from build123d import *

# Parameters (mm, degrees)
SKETCH1_W           = 60
SKETCH1_H           = 160
SKETCH1_R           = 10
SKETCH1_R_2         = 10.5
BOSS_EXTRUDE1_DEPTH = 12
CUT_EXTRUDE1_REACH  = 88.279
SKETCH2_R           = 4
CUT_EXTRUDE2_REACH  = 102.717
SKETCH3_R           = 3


with BuildPart() as part:
    # Sketch1 → Boss-Extrude1 (new body)
    with BuildSketch(Plane(origin=(0, 0, 0), x_dir=(1, 0, 0), z_dir=(0, 1, 0))):
        Rectangle(SKETCH1_W, SKETCH1_H)
        with Locations(Location((0, 0, 0), (0, 0, 270))):
            Circle(SKETCH1_R, mode=Mode.SUBTRACT)
        with Locations(Location((0, 40, 0), (0, 0, 270))):
            Circle(SKETCH1_R_2, mode=Mode.SUBTRACT)
        with Locations(Location((0, -40, 0), (0, 0, 270))):
            Circle(SKETCH1_R_2, mode=Mode.SUBTRACT)
    extrude(amount=BOSS_EXTRUDE1_DEPTH)

    # Sketch2 → Cut-Extrude1 (cut, up to next)
    with BuildSketch(Plane(origin=(0, 12, 0), x_dir=(1, 0, 0), z_dir=(0, 1, 0)), mode=Mode.PRIVATE) as cut_extrude1_sk1:
        with Locations(Location((18, 50, 0), (0, 0, 270))):
            Circle(SKETCH2_R)
    cut_extrude1_tool1 = extrude(cut_extrude1_sk1.sketch, amount=-CUT_EXTRUDE1_REACH, mode=Mode.PRIVATE) & part.part
    # Sketch2 → Cut-Extrude1 (cut, up to next)
    with BuildSketch(Plane(origin=(0, 12, 0), x_dir=(1, 0, 0), z_dir=(0, 1, 0)), mode=Mode.PRIVATE) as cut_extrude1_sk2:
        with Locations(Location((18, -50, 0), (0, 0, 270))):
            Circle(SKETCH2_R)
    cut_extrude1_tool2 = extrude(cut_extrude1_sk2.sketch, amount=-CUT_EXTRUDE1_REACH, mode=Mode.PRIVATE) & part.part
    # Sketch2 → Cut-Extrude1 (cut, up to next)
    with BuildSketch(Plane(origin=(0, 12, 0), x_dir=(1, 0, 0), z_dir=(0, 1, 0)), mode=Mode.PRIVATE) as cut_extrude1_sk3:
        with Locations(Location((18, -20, 0), (0, 0, 270))):
            Circle(SKETCH2_R)
    cut_extrude1_tool3 = extrude(cut_extrude1_sk3.sketch, amount=-CUT_EXTRUDE1_REACH, mode=Mode.PRIVATE) & part.part
    # Sketch2 → Cut-Extrude1 (cut, up to next)
    with BuildSketch(Plane(origin=(0, 12, 0), x_dir=(1, 0, 0), z_dir=(0, 1, 0)), mode=Mode.PRIVATE) as cut_extrude1_sk4:
        with Locations(Location((18, 20, 0), (0, 0, 270))):
            Circle(SKETCH2_R)
    cut_extrude1_tool4 = extrude(cut_extrude1_sk4.sketch, amount=-CUT_EXTRUDE1_REACH, mode=Mode.PRIVATE) & part.part
    add(cut_extrude1_tool1.solids().sort_by_distance((18, 12, -50))[0], mode=Mode.SUBTRACT)
    add(cut_extrude1_tool2.solids().sort_by_distance((18, 12, 50))[0], mode=Mode.SUBTRACT)
    add(cut_extrude1_tool3.solids().sort_by_distance((18, 12, 20))[0], mode=Mode.SUBTRACT)
    add(cut_extrude1_tool4.solids().sort_by_distance((18, 12, -20))[0], mode=Mode.SUBTRACT)

    # Sketch3 → Cut-Extrude2 (cut, up to next)
    with BuildSketch(Plane(origin=(30, 0, 0), x_dir=(0, 0, -1), z_dir=(1, 0, 0)), mode=Mode.PRIVATE) as cut_extrude2_sk1:
        with Locations((50, 6)):
            Circle(SKETCH3_R)
    cut_extrude2_tool1 = extrude(cut_extrude2_sk1.sketch, amount=-CUT_EXTRUDE2_REACH, mode=Mode.PRIVATE) & part.part
    # Sketch3 → Cut-Extrude2 (cut, up to next)
    with BuildSketch(Plane(origin=(30, 0, 0), x_dir=(0, 0, -1), z_dir=(1, 0, 0)), mode=Mode.PRIVATE) as cut_extrude2_sk2:
        with Locations((20, 6)):
            Circle(SKETCH3_R)
    cut_extrude2_tool2 = extrude(cut_extrude2_sk2.sketch, amount=-CUT_EXTRUDE2_REACH, mode=Mode.PRIVATE) & part.part
    # Sketch3 → Cut-Extrude2 (cut, up to next)
    with BuildSketch(Plane(origin=(30, 0, 0), x_dir=(0, 0, -1), z_dir=(1, 0, 0)), mode=Mode.PRIVATE) as cut_extrude2_sk3:
        with Locations((-20, 6)):
            Circle(SKETCH3_R)
    cut_extrude2_tool3 = extrude(cut_extrude2_sk3.sketch, amount=-CUT_EXTRUDE2_REACH, mode=Mode.PRIVATE) & part.part
    # Sketch3 → Cut-Extrude2 (cut, up to next)
    with BuildSketch(Plane(origin=(30, 0, 0), x_dir=(0, 0, -1), z_dir=(1, 0, 0)), mode=Mode.PRIVATE) as cut_extrude2_sk4:
        with Locations((-50, 6)):
            Circle(SKETCH3_R)
    cut_extrude2_tool4 = extrude(cut_extrude2_sk4.sketch, amount=-CUT_EXTRUDE2_REACH, mode=Mode.PRIVATE) & part.part
    add(cut_extrude2_tool1.solids().sort_by_distance((30, 6, -50))[0], mode=Mode.SUBTRACT)
    add(cut_extrude2_tool2.solids().sort_by_distance((30, 6, -20))[0], mode=Mode.SUBTRACT)
    add(cut_extrude2_tool3.solids().sort_by_distance((30, 6, 20))[0], mode=Mode.SUBTRACT)
    add(cut_extrude2_tool4.solids().sort_by_distance((30, 6, 50))[0], mode=Mode.SUBTRACT)


solid = part.part
Check sheet for the modelled part. Datum: model origin and axes. Units: mm. A direction names the side the tool comes from. Coordinates: 2 decimals unless noted, no trailing zeros. Loops run counter-clockwise (first coordinate to the right, second up) from the corner with the lowest first, then second, coordinate; pieces in that order, holes last. Notation, with made-up numbers: (9.5, 65.25) -> (51.5, 65.25) arc R19 ccw to (51.5, 88.25) -> close; hole circle Ø1 at (58.5, 66). An arc over 180 degrees is marked (long way). Write item = value, one per line. Start each with the question number.
1. Material ranges on line 1 (Z direction, x = 25, y = 6); line 2 (Z direction, x = 20, y = 3); line 3 (X direction, y = 2.5, z = -40), recorded low to high.
2. Section check B-B on z = 0. Record the cut outline in (x, y).
3. Depth check by flat-ended pin: P1, Ø17, axis at x = 0, z = 40, coming from the +Y side; P2, Ø5, axis at y = 6, z = -50, coming from the +X side. Enter the tip coordinate at first touch or a pass-through.
4. Section check A-A on z = -20. Record the cut outline in (x, y).
5. Tool access check on faces 4 (the cylindrical face through (-9.76, 5.92, -2.17)), 5 (the cylindrical face through (25.39, 3.07, -49.35)). Record the directions out of +Z, -Z, +X, -X, +Y, -Y that give a thin tool (end or side, any length) a straight path to the whole face; none if there is none.
6. Section check C-C on z = -39.5. Record the cut outline in (x, y), then the cut area to 3 significant figures.
7. Draft check along X on faces 1 (the flat face through (-14, 0, -1)), 2 (the flat face through (30, 6, 1)), 3 (the cylindrical face through (14.095, 6.084, 19.133)). Enter one of: released by +X, released by -X, zero draft, split by the parting line, or undercut.
Responses:
q1.line_1 = -80 to -53, -47 to -23, -17 to 17, 23 to 47, 53 to 80
q1.line_2 = -80 to -53.46, -46.54 to -23.46, -16.54 to 16.54, 23.46 to 46.54, 53.46 to 80
q1.line_3 = -30 to -10.5, 10.5 to 30
q2.outline = (-30, 0) -> (-10, 0) -> (-10, 12) -> (-30, 12) -> close; (10, 0) -> (30, 0) -> (30, 12) -> (10, 12) -> close
q3.P1 = through
q3.P2 = 14.88
q4.outline = (-30, 0) -> (14, 0) -> (14, 12) -> (-30, 12) -> close; (22, 0) -> (30, 0) -> (30, 3) -> (22, 3) -> close; (22, 9) -> (30, 9) -> (30, 12) -> (22, 12) -> close
q5.face_4 = +Y, -Y
q5.face_5 = +X
q6.outline = (-30, 0) -> (-10.49, 0) -> (-10.49, 12) -> (-30, 12) -> close; (10.49, 0) -> (30, 0) -> (30, 12) -> (10.49, 12) -> close
q6.area = 468 mm2
q7.face_1 = zero draft
q7.face_2 = released by +X
q7.face_3 = undercut
